```python
from build123d import *

# Parameters (mm, degrees)
F1_DEPTH = 18


with BuildPart() as f1:
    # F0 (on Front) → F1 (new body)
    with BuildSketch(Plane.XZ):
        Polygon((-199, -149), (-99, -149), (99, -149), (99, -51), (99, 149), (-99, 149), (-99, -51), (-199, -51), align=None)
        Polygon((-99, 149), (-199, -51), (-99, -51), align=None)
    extrude(amount=F1_DEPTH)


solid = f1.part
```
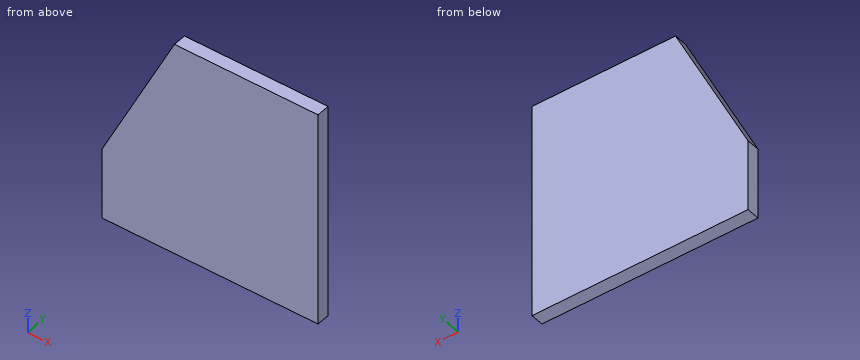
Source: CAD feature listing. Evaluate the final solid. Frame: model axes, mm. Round coordinates to 2 decimals unless told otherwise and drop trailing zeros. Loops run counter-clockwise (first coordinate to the right, second up) from the corner with the lowest first, then second, coordinate; pieces in that order, holes last. Notation, with made-up numbers: M 78,-4.75 L 123,-4.75 A18 ccw 123,28.25 Z; hole C 48.25,28 d6. An arc over 180 degrees is marked long. Use a Markdown table: item, result. Add a question column.
1. Cut plane B-B, the plane x = -180. Output: boundary loops of the cut face in (y, z).
2. Cut plane C-C, the plane z = 93. Output: boundary loops of the cut face in (x, y), and give its area (3 significant figures).
3. Contact query for flat-ended pins moving along their axis: pin 1 (8 mm diameter, centred on y = -3, z = -42, fed in from -X); pin 2 (3 mm diameter, centred on y = -11.5, z = 96, fed in from -X); pin 3 (5 mm diameter, centred on y = -14, z = 20.5, fed in from -X). Output: stop coordinate, or through.
4. Cut plane A-A, the plane y = -5.75. Output: boundary loops of the cut face in (x, z).
5. Ray query, line 1 along X through (y, z) = (-2.75, 64.5); line 2 along X through (y, z) = (-3.25, 136); line 3 along Z through (x, y) = (-170, -7.25). Return the intervals inside material, ascending. Write a range as [from, to].
Solution:
| question | item | result |
|---|---|---|
| 1 | outline | M -18,-149 L 0,-149 L 0,-13 L -18,-13 Z |
| 2 | outline | M -127,-18 L 99,-18 L 99,0 L -127,0 Z |
| 2 | area | 4,070 mm2 |
| 3 | pin 1 | stops at x = -196.5 |
| 3 | pin 2 | stops at x = -126.25 |
| 3 | pin 3 | stops at x = -164.5 |
| 4 | outline | M -199,-149 L 99,-149 L 99,149 L -99,149 L -199,-51 Z |
| 5 | line 1 | x = [-141.25, 99] |
| 5 | line 2 | x = [-105.5, 99] |
| 5 | line 3 | z = [-149, 7] |
